```python
from build123d import *

# Parameters (mm, degrees)
SKETCH4_W                                      = 24.13
SKETCH4_H                                      = 0.8255
CUT_EXTRUDE1_DEPTH                             = 49.057945385
SKETCH5_W                                      = 34.925
SKETCH5_H                                      = 0.8255
CUT_EXTRUDE2_DEPTH                             = 49.057945385
F_6_32_TAPPED_HOLE1_AT_2_COUNT                 = 2
F_6_32_TAPPED_HOLE1_AT_2_PITCH                 = 6.35
F_6_32_TAPPED_HOLE1_AT_3_COUNT                 = 2
F_6_32_TAPPED_HOLE1_AT_3_PITCH                 = 17.4625
F_6_32_TAPPED_HOLE1_AT_4_COUNT                 = 2
F_6_32_TAPPED_HOLE1_AT_4_PITCH                 = 23.8125
CBORE_FOR_6_SOCKET_HEAD_CAP_SCREW1_D           = 3.7973
CBORE_FOR_6_SOCKET_HEAD_CAP_SCREW1_DEPTH       = 11.8745
CBORE_FOR_6_SOCKET_HEAD_CAP_SCREW1_CBORE_D     = 7.14502
CBORE_FOR_6_SOCKET_HEAD_CAP_SCREW1_CBORE_DEPTH = 9.8552


with BuildPart() as part:
    # Sketch1 → Revolve1 (revolve)
    with BuildSketch(Plane(origin=(0, 0, 0), x_dir=(1, 0, 0), z_dir=(0, 1, 0))):
        Polygon((3.175, 44.927025994), (3.175, 29.052025994), (4, 29.052025994), (4, 10.002025994), (12.065, 10.002025994), (12.065, 44.927025994), align=None)
    revolve(axis=Axis((0, 0, 0), (0, 0, -1)))

    # Sketch4 → Cut-Extrude1 (cut, through all)
    with BuildSketch(Plane(origin=(0, 0, 0), x_dir=(1, 0, 0), z_dir=(0, 1, 0))):
        with Locations((0, 28.639275994)):
            Rectangle(SKETCH4_W, SKETCH4_H)
    extrude(amount=CUT_EXTRUDE1_DEPTH, mode=Mode.SUBTRACT)

    # Sketch5 → Cut-Extrude2 (cut, through all)
    with BuildSketch(Plane(origin=(0, 0, 0), x_dir=(0, 0, -1), z_dir=(1, 0, 0))):
        with Locations((27.464525994, 0.41275)):
            Rectangle(SKETCH5_W, SKETCH5_H)
    extrude(amount=CUT_EXTRUDE2_DEPTH, mode=Mode.SUBTRACT)

    # Sketch6 → #6-32 Tapped Hole1 (revolve, cut)
    with BuildSketch(Plane(origin=(8.0325, 0, -16.352025994), x_dir=(0, 0, 1), z_dir=(1, 0, 0))):
        Polygon((0, 0), (0, 11.98869403), (1.35255, 11.176), (1.35255, 0), align=None)
    f_6_32_tapped_hole1 = revolve(axis=Axis((8.0325, 6.35, -16.352025994), (0, -1, 0)), mode=Mode.SUBTRACT)

    # #6-32 Tapped Hole1 at 2: #6-32 Tapped Hole1 ×2
    with Locations(*[(0, 0, -i * F_6_32_TAPPED_HOLE1_AT_2_PITCH) for i in range(1, F_6_32_TAPPED_HOLE1_AT_2_COUNT)]):
        add(f_6_32_tapped_hole1, mode=Mode.SUBTRACT)

    # #6-32 Tapped Hole1 at 3: #6-32 Tapped Hole1 ×2
    with Locations(*[(0, 0, -i * F_6_32_TAPPED_HOLE1_AT_3_PITCH) for i in range(1, F_6_32_TAPPED_HOLE1_AT_3_COUNT)]):
        add(f_6_32_tapped_hole1, mode=Mode.SUBTRACT)

    # #6-32 Tapped Hole1 at 4: #6-32 Tapped Hole1 ×2
    with Locations(*[(0, 0, -i * F_6_32_TAPPED_HOLE1_AT_4_PITCH) for i in range(1, F_6_32_TAPPED_HOLE1_AT_4_COUNT)]):
        add(f_6_32_tapped_hole1, mode=Mode.SUBTRACT)

    # CBORE for #6 Socket Head Cap Screw1
    with Locations(Plane(origin=(0, 12.7, 0), x_dir=(-1, 0, 0), z_dir=(0, 1, 0))):
        with Locations((-8.0325, -16.352025994), (-8.0325, -22.702025994), (-8.0325, -33.814525994), (-8.0325, -40.164525994)):
            CounterBoreHole(CBORE_FOR_6_SOCKET_HEAD_CAP_SCREW1_D / 2, CBORE_FOR_6_SOCKET_HEAD_CAP_SCREW1_CBORE_D / 2, CBORE_FOR_6_SOCKET_HEAD_CAP_SCREW1_CBORE_DEPTH, depth=CBORE_FOR_6_SOCKET_HEAD_CAP_SCREW1_DEPTH)


solid = part.part
```
Geometry: final body of the model. Coordinates: model frame, mm. A direction names the side the tool comes from. Round coordinates to 2 decimals unless told otherwise and drop trailing zeros. Order: outer loops, then holes, each group sorted by start corner. A loop starts at its lowest first (then second) coordinate and runs counter-clockwise, first axis right, second up. Notation, with made-up numbers: M -4,85.5 L 53,85.5 A9 cw 53,97.5 Z; hole C -8.75,-2.75 d11. An arc over 180 degrees is marked long. Use one line per item in the form item = value. Start each with the question number.
Q1. Mould query, pull axis Z, two halves, no side actions, for faces 1 (the face through (3, -3, -10.002)), 2 (the face through (8, 0.826, -19)), 3 (the face through (7.79, 1.82, -38.28)). Classes: +Z half, -Z half, draft (parallel to the pull), parting line (faces both ways), or undercut.
Q2. Access query for faces 4 (the face through (-8.68, -8.38, -27.71)), 5 (the face through (0, 6, -28.227)), 6 (the face through (6.69, -4.95, -40.34)), 7 (the face through (9.05, 1.82, -14.75)), 8 (the face through (-3.957, -0.584, -19.394)). Directions: +Z, -Z, +X, -X, +Y, -Y. A direction counts if a zero-diameter tool reaches every point of the face in a straight line with its end or side. Return the directions, or none.
Q3. Cut plane A-A (y = -2.5). Return loops of the section in (x, z).
Q4. Cut plane C-C (z = -15.5). Return loops of the section in (x, y) (1 decimal), and give its area (3 significant figures).
Q5. Cut plane B-B (x = 0). Return loops of the section in (y, z) (3 decimals), and give its area (3 significant figures).
Q6. Material intervals for line 1 (Z direction, x = -8.5, y = 5.5); line 2 (Z direction, x = 7.5, y = 3); line 3 (Z direction, x = 8.5, y = 1.5), sorted ascending. Write a range as [from, to].
Q7. Pin query (flat end, axial travel): pin 1 Ø8 at (x, z) = (8.03, -33.81) entering from +Y; pin 2 Ø4 at (x, z) = (7, -22.5) entering from -Y; pin 3 Ø12 at (y, z) = (-2, -20.5) entering from -X (3 decimals); pin 4 Ø4 at (y, z) = (-8, -36.5) entering from +X. Return the tip coordinate at first contact, or that it passes through.
Q8. Cut plane D-D (y = -7.5). Return loops of the section in (x, z), and give its area (3 significant figures).
Geometry results:
q1.face_1 = +Z half
q1.face_2 = draft
q1.face_3 = undercut
q2.face_4 = +Z, -Z
q2.face_5 = +X, -X, +Y
q2.face_6 = +Y, -Y
q2.face_7 = +Y
q2.face_8 = +Z
q3.outline = M -11.8,-44.93 L -1.96,-44.93 L -1.96,-29.05 L -3.12,-29.05 L -3.12,-10 L -11.8,-10 Z; M 1.96,-44.93 L 11.8,-44.93 L 11.8,-10 L 3.12,-10 L 3.12,-29.05 L 1.96,-29.05 Z; hole C 8.03,-40.16 d2.71; hole C 8.03,-33.81 d2.71; hole C 8.03,-22.7 d2.71; hole C 8.03,-16.35 d2.71
q4.outline = M 3.9,0.8 L 6.3,0.8 L 6.3,2.8 L 4.6,2.8 L 4.6,11.2 A12.1 ccw long 7,-9.8 L 7,0 L 4,0 A4 cw long Z; M 9.1,-7.9 A12.1 ccw 12.1,0 L 9.1,0 Z; M 9.7,0.8 L 12,0.8 A12.1 ccw 11.5,3.6 L 11.5,2.8 L 9.7,2.8 Z
q4.area = 335 mm^2
q5.outline = M -12.065,-44.927 L -3.175,-44.927 L -3.175,-29.052 L -4,-29.052 L -4,-10.002 L -12.065,-10.002 Z; M 3.175,-44.927 L 12.065,-44.927 L 12.065,-29.052 L 3.175,-29.052 Z; M 4,-28.227 L 12.065,-28.227 L 12.065,-10.002 L 4,-10.002 Z
q5.area = 583 mm^2
q6.line_1 = [-44.93, -29.05], [-28.23, -10]
q6.line_2 = [-44.93, -43.7], [-30.28, -29.05], [-28.23, -26.23], [-12.82, -10]
q6.line_3 = [-44.93, -42], [-38.32, -35.65], [-31.97, -29.05], [-28.23, -24.54], [-20.86, -18.19], [-14.51, -10]
q7.pin_1 = 11.37
q7.pin_2 = -10.98
q7.pin_3 = -12.065
q7.pin_4 = 10.47
q8.outline = M -9.45,-44.93 L 9.45,-44.93 L 9.45,-10 L -9.45,-10 Z; hole C 8.03,-40.16 d2.71; hole C 8.03,-33.81 d2.71; hole C 8.03,-22.7 d2.71; hole C 8.03,-16.35 d2.71
q8.area = 637 mm^2
